Could you check a few things on this model? Use its own coordinates, in mm. Give positions to 0.01 mm unless a question says otherwise; leave off trailing zeros. Loops run counter-clockwise (first coordinate to the right, second up) from the corner with the lowest first, then second, coordinate; pieces in that order, holes last. Notation, with made-up numbers: (26.5, -39) - (49.5, -39) arc R30 ccw to (49.5, -12) - close; hole circle Ø5 at (71, 65.25). An arc over 180 degrees is marked (long way). Write each question's results on one line, items separated by ' | '. Start each with the question number.
(1) For pin 1 (2 mm diameter, centred on y = -0.5, z = -86, fed in from -X); pin 2 (1.6 mm diameter, centred on x = 120, y = -1.5, fed in from -Z); pin 3 (1 mm diameter, centred on x = -85.5, y = -2.5, fed in from -Z); pin 4 (1 mm diameter, centred on x = -83.5, z = -87.5, fed in from +Y) (3 decimals), each with a flat end and sliding along its axis, tell me the tip position at first contact or that it passes through.
(2) Suppose I cut it at A-A (y = -1.05). Please give me the cut outline in (x, z).
(3) Suppose I cut it at B-B (z = -13). Please give me the cut outline in (x, y) (3 decimals), and give its area (3 significant figures).
(4) I need wall thicknesses on line 1 (X direction, y = -2.75, z = -44); line 2 (X direction, y = -1.7, z = -20). Which ranges of each line are inside material? Lowest first, please.
from build123d import *

# Parameters (mm, degrees)
F0_W     = 210
F0_H     = 40
F1_DEPTH = 4
F2_W     = 2
F2_H     = 2.005
F3_DEPTH = 140
F4_W     = 2
F4_H     = 1.995
F5_DEPTH = 10
F6_W     = 2
F6_H     = 1.995
F7_DEPTH = 10


with BuildPart() as f1:
    # F0 (on Front) → F1 (new body)
    with BuildSketch(Plane.XZ):
        with Locations((18.386809, 24.299242)):
            Rectangle(F0_W, F0_H)
    extrude(amount=F1_DEPTH)

    # F2 (on face) → F3 (join)
    with BuildSketch(Plane(origin=(0, 0, 4.299242), x_dir=(1, 0, 0), z_dir=(0, 0, -1))):
        with Locations((-83.608191, 2.9975)):
            Rectangle(F2_W, F2_H)
        Polygon((-82.608191, 4), (-82.608191, 1.995), (-82.608191, 0), (119.381809, 0), (119.381809, 1.995), (119.381809, 4), align=None)
        with Locations((120.381809, 2.9975)):
            Rectangle(F2_W, F2_H)
    extrude(amount=F3_DEPTH)

    # F4 (on face) → F5 (join)
    with BuildSketch(Plane(origin=(0, 0, 4.299242), x_dir=(1, 0, 0), z_dir=(0, 0, -1))):
        with Locations((120.381809, 0.9975)):
            Rectangle(F4_W, F4_H)
    extrude(amount=F5_DEPTH)

    # F6 (on face) → F7 (join)
    with BuildSketch(Plane(origin=(0, 0, 4.299242), x_dir=(1, 0, 0), z_dir=(0, 0, -1))):
        with Locations((-83.608191, 0.9975)):
            Rectangle(F6_W, F6_H)
    extrude(amount=F7_DEPTH)


solid = f1.part
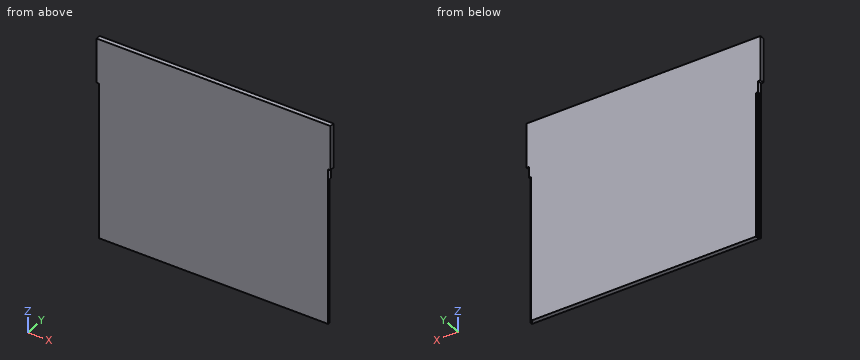
Output values:
1) pin 1: x = -82.61 | pin 2: z = -135.7 | pin 3: z = 4.3 | pin 4: y = -1.995
2) outline: (-86.61, 4.3) - (-84.61, 4.3) - (-84.61, -5.7) - (-82.61, -5.7) - (-82.61, -135.7) - (119.38, -135.7) - (119.38, -5.7) - (121.38, -5.7) - (121.38, 4.3) - (123.39, 4.3) - (123.39, 44.3) - (-86.61, 44.3) - close
3) outline: (-84.608, -4) - (121.382, -4) - (121.382, -1.995) - (119.382, -1.995) - (119.382, 0) - (-82.608, 0) - (-82.608, -1.995) - (-84.608, -1.995) - close | area: 816 mm2
4) line 1: -84.61 to 121.38 | line 2: -82.61 to 119.38
